```python
from build123d import *

# Parameters (mm, degrees)
SKETCH1_W           = 45
SKETCH1_H           = 40
SKETCH1_R           = 1.8
SKETCH1_R_2         = 1.75
SKETCH1_R_3         = 1.7
SKETCH1_R_4         = 3.2
SKETCH1_R_5         = 3.15
SKETCH1_R_6         = 3.1
BOSS_EXTRUDE1_DEPTH = 5
SKETCH2_W           = 8
SKETCH2_H           = 40
BOSS_EXTRUDE2_DEPTH = 10
CUT_EXTRUDE1_REACH  = 53.478
CHAMFER1_SIZE       = 5
CHAMFER2_SIZE       = 5
CHAMFER2_SIZE2      = 5.958767963
CHAMFER3_SIZE       = 5
CHAMFER4_SIZE       = 5
CHAMFER4_SIZE2      = 7.140740034
CHAMFER5_SIZE       = 5
CHAMFER5_SIZE2      = 4.195498156


with BuildPart() as part:
    # Sketch1 → Boss-Extrude1 (new body)
    with BuildSketch(Plane.XY):
        with Locations((-7.5, 0)):
            Rectangle(SKETCH1_W, SKETCH1_H)
        with Locations((-20, 0)):
            Circle(SKETCH1_R, mode=Mode.SUBTRACT)
        with Locations((-10, 0)):
            Circle(SKETCH1_R_2, mode=Mode.SUBTRACT)
        Circle(SKETCH1_R_3, mode=Mode.SUBTRACT)
        with Locations((-20, 10)):
            Circle(SKETCH1_R_4, mode=Mode.SUBTRACT)
        with Locations((-10, 10)):
            Circle(SKETCH1_R_5, mode=Mode.SUBTRACT)
        with Locations((0, 10)):
            Circle(SKETCH1_R_6, mode=Mode.SUBTRACT)
        Polygon((-16.304958277, -10), (-18.152479139, -6.8), (-21.847520861, -6.8), (-23.695041723, -10), (-21.847520861, -13.2), (-18.152479139, -13.2), align=None, mode=Mode.SUBTRACT)
        Polygon((-6.362693304, -10), (-8.181346652, -6.85), (-11.818653348, -6.85), (-13.637306696, -10), (-11.818653348, -13.15), (-8.181346652, -13.15), align=None, mode=Mode.SUBTRACT)
        Polygon((3.579571669, -10), (1.789785834, -6.9), (-1.789785834, -6.9), (-3.579571669, -10), (-1.789785834, -13.1), (1.789785834, -13.1), align=None, mode=Mode.SUBTRACT)
    extrude(amount=BOSS_EXTRUDE1_DEPTH)

    # Sketch2 → Boss-Extrude2 (add)
    with BuildSketch(Plane.XY.offset(5)):
        with Locations((11, 0)):
            Rectangle(SKETCH2_W, SKETCH2_H)
    extrude(amount=BOSS_EXTRUDE2_DEPTH)

    # Sketch3 → Cut-Extrude1 (cut, up to next)
    with BuildSketch(Plane(origin=(15, 0, 0), x_dir=(0, 0, -1), z_dir=(1, 0, 0)), mode=Mode.PRIVATE) as cut_extrude1_sk1:
        with BuildLine():
            Line((-11.092738936, 11.302275553), (-11.7, 10.792723019))
            Line((-11.7, 10.792723019), (-11.7, 9.207276981))
            Line((-11.7, 9.207276981), (-11.092738936, 8.697724447))
            ThreePointArc((-11.092738936, 8.697724447), (-8.3, 10), (-11.092738936, 11.302275553))
        make_face()
    cut_extrude1_tool1 = extrude(cut_extrude1_sk1.sketch, amount=-CUT_EXTRUDE1_REACH, mode=Mode.PRIVATE) & part.part
    # Sketch3 → Cut-Extrude1 (cut, up to next)
    with BuildSketch(Plane(origin=(15, 0, 0), x_dir=(0, 0, -1), z_dir=(1, 0, 0)), mode=Mode.PRIVATE) as cut_extrude1_sk2:
        with BuildLine():
            Line((-11.124878317, 1.340577775), (-11.75, 0.816038402))
            Line((-11.75, 0.816038402), (-11.75, -0.816038402))
            Line((-11.75, -0.816038402), (-11.124878317, -1.340577775))
            ThreePointArc((-11.124878317, -1.340577775), (-8.25, 0), (-11.124878317, 1.340577775))
        make_face()
    cut_extrude1_tool2 = extrude(cut_extrude1_sk2.sketch, amount=-CUT_EXTRUDE1_REACH, mode=Mode.PRIVATE) & part.part
    # Sketch3 → Cut-Extrude1 (cut, up to next)
    with BuildSketch(Plane(origin=(15, 0, 0), x_dir=(0, 0, -1), z_dir=(1, 0, 0)), mode=Mode.PRIVATE) as cut_extrude1_sk3:
        with BuildLine():
            Line((-11.157017697, -8.621120002), (-11.8, -9.160646215))
            Line((-11.8, -9.160646215), (-11.8, -10.839353785))
            Line((-11.8, -10.839353785), (-11.157017697, -11.378879998))
            ThreePointArc((-11.157017697, -11.378879998), (-8.2, -10), (-11.157017697, -8.621120002))
        make_face()
    cut_extrude1_tool3 = extrude(cut_extrude1_sk3.sketch, amount=-CUT_EXTRUDE1_REACH, mode=Mode.PRIVATE) & part.part
    add(cut_extrude1_tool1.solids().sort_by_distance((15, 10, 10.029483))[0], mode=Mode.SUBTRACT)
    add(cut_extrude1_tool2.solids().sort_by_distance((15, 0, 10.03035))[0], mode=Mode.SUBTRACT)
    add(cut_extrude1_tool3.solids().sort_by_distance((15, -10, 10.031217))[0], mode=Mode.SUBTRACT)

    # Chamfer1
    chamfer1_edges = [part.edges().sort_by_distance(p)[0] for p in [
        (-30, -20, 2.5),
        (-30, 20, 2.5),
        (11, -20, 15),
        (11, 20, 15),
    ]]
    chamfer(chamfer1_edges, length=CHAMFER1_SIZE)

    # Chamfer2
    chamfer2_edges = [part.edges().sort_by_distance(p)[0] for p in [
        (-5, 20, 0),
    ]]
    chamfer2_side = [part.faces().sort_by_distance(p)[0] for p in [
        (-6.76599085, 0.061969604, 0),
    ]]
    chamfer(chamfer2_edges, length=CHAMFER2_SIZE, length2=CHAMFER2_SIZE2, reference=chamfer2_side[0])

    # Chamfer3
    chamfer3_edges = [part.edges().sort_by_distance(p)[0] for p in [
        (-5, -20, 0),
    ]]
    chamfer(chamfer3_edges, length=CHAMFER3_SIZE)

    # Chamfer4
    chamfer4_edges = [part.edges().sort_by_distance(p)[0] for p in [
        (15, 0, 0),
    ]]
    chamfer4_side = [part.faces().sort_by_distance(p)[0] for p in [
        (-6.951751809, 0.085391734, 0),
    ]]
    chamfer(chamfer4_edges, length=CHAMFER4_SIZE, length2=CHAMFER4_SIZE2, reference=chamfer4_side[0])

    # Chamfer5
    chamfer5_edges = [part.edges().sort_by_distance(p)[0] for p in [
        (-30, 0, 0),
    ]]
    chamfer5_side = [part.faces().sort_by_distance(p)[0] for p in [
        (-10, -14.5, 0),
    ]]
    chamfer(chamfer5_edges, length=CHAMFER5_SIZE, length2=CHAMFER5_SIZE2, reference=chamfer5_side[0])


solid = part.part
```
Could you check a few things on this model? Use its own coordinates, in mm. A direction names the side the tool comes from. Round coordinates to 2 decimals unless told otherwise and drop trailing zeros. Write each loop counter-clockwise with the first axis right and the second up, starting at its lowest first coordinate (ties: lowest second). Pieces come first, ordered by that corner, then holes. Notation, with made-up numbers: M 83.5,21 L 125.5,21 A37 cw 125.5,57 Z; hole C -29.5,45 d3. An arc over 180 degrees is marked long. Write each question's results on one line, items separated by ' | '. Start each with the question number.
1. On a 3-axis mill with a long thin cutter (end or side, diameter ignored), from which of +Z, -Z, +X, -X, +Y, -Y can I reach the whole of each face in a straight line? I mean faces 4 (the face through (-22.76, -8.38, 2.46)), 5 (the face through (-27.5, -0.3, 2.1)), 6 (the face through (7, 0, 8)). Say none if no direction works.
2. Imagine slicing it at A-A on y = 10. List the corners of the cut face in (x, z) for me, and give its area (3 significant figures).
3. I'm going to push flat-ended pins straight in: pin 1 Ø8 at (x, y) = (0, 10) entering from +Z; pin 2 Ø1 at (y, z) = (1.5, 9) entering from -X; pin 3 Ø1.3 at (x, y) = (13, 10) entering from -Z. Where does each tip first touch, or does it pass through?
4. Imagine slicing it at D-D on y = 0. List the corners of the cut face in (x, z) for me, and give its area (3 significant figures).
5. Imagine slicing it at B-B on x = 0. List the corners of the cut face in (y, z) for me.
6. I need wall thicknesses on L1, parallel to X at y = 10.5, z = 0.5; L2, parallel to Y at x = 0, z = 3.35; L3, parallel to X at y = 8.5, z = 2. Which ranges of each line are inside material? Lowest first, please. Write a range as from..to.
7. Thinking about a two-plate mould opening in X: for faces 1 (the face through (-2.697, -11.528, 2.465)), 2 (the face through (11, 0, 15)), 3 (the face through (15, 0, 12)), which applies, +X half, -X half, draft (parallel to the pull), parting line (faces both ways), or undercut?
8. Imagine slicing it at C-C on z = 9. List the corners of the cut face in (x, y) for me, and give its area (3 significant figures).
Result sheet:
1) face 4: +Z, -Z | face 5: -Z, -X, +Y, -Y | face 6: +Z, -X, +Y, -Y
2) outline: M -30,4.2 L -25,0 L -23.2,0 L -23.2,5 L -30,5 Z; M -16.8,0 L -13.15,0 L -13.15,5 L -16.8,5 Z; M -6.85,0 L -3.1,0 L -3.1,5 L -6.85,5 Z; M 3.1,0 L 10,0 L 15,7.14 L 15,8.3 L 7,8.3 L 7,5 L 3.1,5 Z; M 7,11.7 L 15,11.7 L 15,15 L 7,15 Z | area: 155 mm^2
3) pin 1: stops at z = 5 | pin 2: stops at x = 7 | pin 3: stops at z = 3.36
4) outline: M -30,4.2 L -25,0 L -21.8,0 L -21.8,5 L -30,5 Z; M -18.2,0 L -11.75,0 L -11.75,5 L -18.2,5 Z; M -8.25,0 L -1.7,0 L -1.7,5 L -8.25,5 Z; M 1.7,0 L 10,0 L 15,7.14 L 15,8.25 L 7,8.25 L 7,5 L 1.7,5 Z; M 7,11.75 L 15,11.75 L 15,15 L 7,15 Z | area: 196 mm^2
5) outline: M -20,5 L -15,0 L -13.1,0 L -13.1,5 Z; M -6.9,0 L -1.7,0 L -1.7,5 L -6.9,5 Z; M 1.7,0 L 6.9,0 L 6.9,5 L 1.7,5 Z; M 13.1,0 L 15,0 L 19.2,5 L 13.1,5 Z
6) L1: x = -25.6..-23.16, -16.84..-13.11, -6.89..-3.06, 3.06..10.35 | L2: y = -18.35..-13.1, -6.9..-1.7, 1.7..6.9, 13.1..17.81 | L3: x = -27.38..-22.83, -17.17..-12.77, -7.23..-2.71, 2.71..11.4
7) face 1: undercut | face 2: draft | face 3: +X half
8) outline: M 7,-20 L 15,-20 L 15,-11.5 L 7,-11.5 Z; M 7,-8.5 L 15,-8.5 L 15,-1.44 L 7,-1.44 Z; M 7,1.44 L 15,1.44 L 15,8.63 L 7,8.63 Z; M 7,11.37 L 15,11.37 L 15,20 L 7,20 Z | area: 251 mm^2
